Source: CAD feature listing. Evaluate the final solid. Frame: model axes, mm. A direction names the side the tool comes from. Give positions to 0.01 mm unless a question says otherwise; leave off trailing zeros. Write each loop counter-clockwise with the first axis right and the second up, starting at its lowest first coordinate (ties: lowest second). Pieces come first, ordered by that corner, then holes. Notation, with made-up numbers: (15, 6.5) -> (65, 6.5) arc R24 ccw to (65, 28.5) -> close; hole circle Ø11 at (22, 60). An arc over 180 degrees is marked (long way). Write item = value, one per line.
from build123d import *

# Parameters (mm, degrees)
SKETCH_1_W          = 60
SKETCH_1_H          = 70
SKETCH_3_R          = 7.5
CUT_EXTRUDE_1_DEPTH = 17


with BuildPart() as part:
    # Эскиз1 → Повернуть1 (revolve)
    with BuildSketch(Plane.XY, mode=Mode.PRIVATE) as revolve_1_sk:
        Polygon((-40, 80), (40, 80), (40, 78), (32, 78), (32, 6), (30, 6), (-30, 6), (-32, 6), (-32, 78), (-40, 78), align=None)
        with Locations((0, 43)):
            Rectangle(SKETCH_1_W, SKETCH_1_H, mode=Mode.SUBTRACT)
    revolve(revolve_1_sk.sketch.rotate(Axis((-118.179588976, 0, 0), (1, 0, 0)), 180), axis=Axis((-118.179588976, 0, 0), (1, 0, 0)))

    # Эскиз3 → Вырез-Вытянуть1 (cut)
    with BuildSketch(Plane.ZY.offset(32)):
        with Locations(Location((0, -49.984788399, 0), (0, 0, 270))):
            Circle(SKETCH_3_R)
    extrude(amount=-CUT_EXTRUDE_1_DEPTH, mode=Mode.SUBTRACT)


solid = part.part
(1) Section query C-C (x = 27). Return loops of the section in (y, z), plus the area to 3 significant figures.
Values follow:
outline = circle Ø160 at (0, 0); circle Ø16 at (0, 0); hole circle Ø156 at (0, 0); hole circle Ø12 at (0, 0)
area = 1,080 mm2
(2) Access query for faces 1 (the face through (-36.056, 10.154, -77.336)), 2 (the face through (0.42, 1.73, 7.81)), 3 (the face through (40, -17, 77)), 4 (the face through (0.448, -5.723, -1.802)), 5 (the face through (32, 1, 16)). Directions: +Z, -Z, +X, -X, +Y, -Y. A direction counts if a zero-diameter tool reaches every point of the face in a straight line with its end or side. Return the directions, or none.
Values follow:
face_1 = -X
face_2 = none
face_3 = +Z, -Z, +X, +Y, -Y
face_4 = +X, -X
face_5 = +X
(3) Section query D-D (y = 52.5). Return loops of the section in (x, z).
Values follow:
outline = (-40, -60.36) -> (40, -60.36) -> (40, -57.69) -> (32, -57.69) -> (32, 57.69) -> (40, 57.69) -> (40, 60.36) -> (-40, 60.36) -> (-40, 57.69) -> (-32, 57.69) -> (-32, -57.69) -> (-40, -57.69) -> close; hole (-30, -57.69) -> (30, -57.69) -> (30, 57.69) -> (-30, 57.69) -> close
(4) Section query B-B (z = 0). Return loops of the section in (x, y).
Values follow:
outline = (-40, -80) -> (40, -80) -> (40, -78) -> (32, -78) -> (32, -6) -> (-32, -6) -> (-32, -42.48) -> (-30, -42.48) -> (-30, -8) -> (30, -8) -> (30, -78) -> (-30, -78) -> (-30, -57.48) -> (-32, -57.48) -> (-32, -78) -> (-40, -78) -> close; (-40, 78) -> (-32, 78) -> (-32, 6) -> (32, 6) -> (32, 78) -> (40, 78) -> (40, 80) -> (-40, 80) -> close; hole (-30, 8) -> (30, 8) -> (30, 78) -> (-30, 78) -> close
(5) First-contact query: pin 1 (6 mm diameter, centred on y = -59, z = 29.5, fed in from -X); pin 2 (4 mm diameter, centred on x = 19, z = -44, fed in from -Y); pin 3 (13.5 mm diameter, centred on y = -49.98, z = 0, fed in from +X); pin 4 (2 mm diameter, centred on x = 3, z = 1, fed in from +Y). Flat tips, straight axial feed; report the tip coordinate or a pass-through.
Values follow:
pin_1 = -32
pin_2 = -68.09
pin_3 = 32
pin_4 = 80
(6) Material intervals for line 1 (X direction, y = 20, z = -51); line 2 (Y direction, x = -22, z = -6.5); line 3 (Z direction, x = -38, y = 0), sorted ascending.
Values follow:
line_1 = -32 to -30, 30 to 32
line_2 = -79.74 to -77.73, -4.66 to 4.66, 77.73 to 79.74
line_3 = -80 to -78, 78 to 80
(7) Pull-direction query (Z, two-part tool) for faces 6 (the face through (-32, 16, -1)), 7 (the face through (0.56, 79.923, -3.517)), 8 (the face through (-40, 77, 17)), 9 (the face through (-30, 16, -1)); classes: pulls with the +Z half, pulls with the -Z half, needs draft (parallel to the pull), parting line crosses it, or undercut.
Values follow:
face_6 = undercut
face_7 = parting line crosses it
face_8 = needs draft
face_9 = undercut
(8) Section query A-A (y = 0). Return loops of the section in (x, z), plus the area to 3 significant figures.
Values follow:
outline = (-40, -80) -> (40, -80) -> (40, -78) -> (32, -78) -> (32, -6) -> (-32, -6) -> (-32, -78) -> (-40, -78) -> close; (-40, 78) -> (-32, 78) -> (-32, 6) -> (32, 6) -> (32, 78) -> (40, 78) -> (40, 80) -> (-40, 80) -> close; hole (-30, -78) -> (30, -78) -> (30, -8) -> (-30, -8) -> close; hole (-30, 8) -> (30, 8) -> (30, 78) -> (-30, 78) -> close
area = 1,140 mm2
